Geometry check sheet. Reference: the model listing, model coordinates, mm. Face numbers are marked on the shaded views. A direction names the side the tool comes from. Give positions to 0.01 mm unless a question says otherwise; leave off trailing zeros. Order: outer loops, then holes, each group sorted by start corner. A loop starts at its lowest first (then second) coordinate and runs counter-clockwise, first axis right, second up. Notation, with made-up numbers: M 69,63 L 81,63 A24 cw 81,74 Z; hole C -30,54.25 d10. An arc over 180 degrees is marked long. Put each result on its own line as item: value. Start each with the question number.
Q1. Section check A-A on x = 0. Record the cut outline in (y, z).
Q2. Access from +Z, -Z, +X, -X, +Y, -Y to the whole of each face (thin tool, end or side, straight path). Record for the marked faces 4 and 5.
Q3. Mould release check, pull along X, two halves, no side actions. Record for the marked faces 1, 2 and 3: +X half, -X half, draft (parallel to the pull), parting line (faces both ways), or undercut.
Q4. Section check B-B on y = 13.75. Record the cut outline in (x, z).
Q5. Material ranges on L1, parallel to Z at x = 2, y = 8.75; L2, parallel to X at y = 11, z = 0; L3, parallel to X at y = 18.2, z = 0, recorded low to high.
Q6. Section check C-C on y = 3. Record the cut outline in (x, z), then the cut area to 3 significant figures.
Q7. Go/stop test with flat-tipped pins: pin 1 (13 mm diameter, centred on x = 0, z = 0, fed in from +Y); pin 2 (8 mm diameter, centred on x = 6, y = 13, fed in from -Z); pin 3 (10 mm diameter, centred on y = 15.5, z = 9, fed in from -X); pin 4 (6 mm diameter, centred on x = -10, y = 14.5, fed in from -Z). Record where each tip stops, or that it passes through.
```python
from build123d import *

# Parameters (mm, degrees)
BOSS_EXTRUDE1_DEPTH     = 20
FILLET1_R               = 1
SKETCH2_R               = 4
CUT_EXTRUDE1_DEPTH      = 15
SKETCH3_R               = 5
CUT_EXTRUDE2_DEPTH      = 15
CUT_EXTRUDE3_DEPTH      = 46.069390988
CUT_EXTRUDE3_DEPTH_BACK = 46.069390988
SKETCH4_R               = 4.1
SKETCH4_R_2             = 3.1


with BuildPart() as part:
    # Sketch1 → Boss-Extrude1 (new body)
    with BuildSketch(Plane(origin=(0, 0, 0), x_dir=(1, 0, 0), z_dir=(0, 1, 0))):
        with BuildLine():
            Line((-9.583148475, 20.357142857), (-19.16629695, -11.785714286))
            ThreePointArc((-19.16629695, -11.785714286), (0, -37.5), (19.16629695, -11.785714286))
            Line((19.16629695, -11.785714286), (9.583148475, 20.357142857))
            ThreePointArc((9.583148475, 20.357142857), (0, 27.5), (-9.583148475, 20.357142857))
        make_face()
    extrude(amount=BOSS_EXTRUDE1_DEPTH)

    # Fillet1
    fillet1_edges = [part.edges().sort_by_distance(p)[0] for p in [
        (0, 20, -27.5),
        (-14.374722712, 20, -4.285714286),
        (0, 20, 37.5),
        (-14.374722712, 0, -4.285714286),
        (0, 0, -27.5),
        (14.374722712, 0, -4.285714286),
        (0, 0, 37.5),
        (14.374722712, 20, -4.285714286),
    ]]
    fillet(fillet1_edges, radius=FILLET1_R)

    # Sketch2 → Cut-Extrude1 (cut)
    with BuildSketch(Plane(origin=(0, 20, 0), x_dir=(1, 0, 0), z_dir=(0, 1, 0))):
        with Locations(Location((0, 15, 0), (0, 0, 270))):
            Circle(SKETCH2_R)
    extrude(amount=-CUT_EXTRUDE1_DEPTH, mode=Mode.SUBTRACT)

    # Sketch3 → Cut-Extrude2 (cut)
    with BuildSketch(Plane.XZ):
        with Locations(Location((0, 0, 0), (0, 0, 270))):
            Circle(SKETCH3_R)
    extrude(amount=-CUT_EXTRUDE2_DEPTH, mode=Mode.SUBTRACT)

    # Sketch4 → Cut-Extrude3 (cut, two sides: drawn at the far end of the back side and taken through both)
    with BuildSketch(Plane.XZ.offset(-15).offset(-CUT_EXTRUDE3_DEPTH_BACK)):
        with Locations(Location((0, 0, 0), (0, 0, 270))):
            Circle(SKETCH4_R)
        with Locations(Location((0, -15, 0), (0, 0, 270))):
            Circle(SKETCH4_R_2)
    extrude(amount=CUT_EXTRUDE3_DEPTH + CUT_EXTRUDE3_DEPTH_BACK, mode=Mode.SUBTRACT)


solid = part.part
```
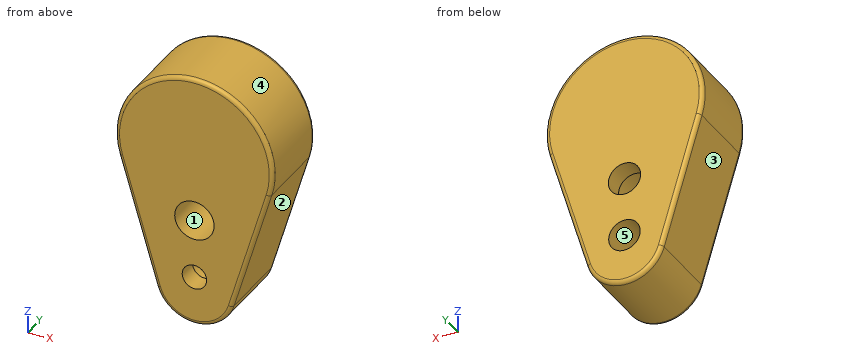
Results found:
1. outline: M 0,-26.5 A1 ccw 1,-27.5 L 19,-27.5 A1 ccw 20,-26.5 L 20,-19 L 5,-19 L 5,-18.1 L 0,-18.1 Z; M 0,-11.9 L 5,-11.9 L 5,-11 L 20,-11 L 20,-4.1 L 15,-4.1 L 15,-5 L 0,-5 Z; M 0,5 L 15,5 L 15,4.1 L 20,4.1 L 20,36.5 A1 ccw 19,37.5 L 1,37.5 A1 ccw 0,36.5 Z
2. face 4: +Y, -Y
2. face 5: +Y
3. face 1: undercut
3. face 2: +X half
3. face 3: -X half
4. outline: M -19.17,11.79 L -9.58,-20.36 A10 ccw 9.58,-20.36 L 19.17,11.79 A20 ccw long Z; hole C 0,0 d10; hole C 0,-15 d8
5. L1: z = -27.3 to -18.46, -11.54 to -4.58, 4.58 to 37.4
5. L2: x = -15.65 to -5, 5 to 15.65
5. L3: x = -15.65 to -4.1, 4.1 to 15.65
6. outline: M -19.17,11.79 L -9.58,-20.36 A10 ccw 9.58,-20.36 L 19.17,11.79 A20 ccw long Z; hole C 0,0 d10; hole C 0,-15 d6.2
6. area: 1,770 mm^2
7. pin 1: stops at y = 20
7. pin 2: stops at z = -27.3
7. pin 3: stops at x = -19.69
7. pin 4: stops at z = -24.64
